Build history of the part. All positions in model axes, mm. Face numbers are marked on the shaded views. Give positions to 0.01 mm unless a question says otherwise; leave off trailing zeros. Return JSON: item names as keys, results as strings. Group by question number.
1) Drill centre lines: probe 1 along Y at (x, z) = (2.8, 3.5) (3 decimals); probe 2 along Z at (x, y) = (3.3, -1.25); probe 3 along X at (y, z) = (0, 1.5). Where is each one in solid material? Low to high. Write a range as from..to.
2) Mould opens along Y. For the marked faces 1, 2 and 3 say: released by +Y, released by -Y, zero draft, split by the parting line, or undercut.
3) Drop a flat-ended pin along its axis: pin 1 (3 mm diameter, centred on y = -2, z = 3.5, fed in from -X). Give the stop position or say it passes through.
```python
from build123d import *

# Parameters (mm, degrees)
BOSS_EXTRUDE1_DEPTH = 6.05
FILLET1_R           = 0.5
FILLET2_R           = 0.1


with BuildPart() as part:
    # Sketch1 → Boss-Extrude1 (new body)
    with BuildSketch(Plane.XY):
        with BuildLine():
            Line((2.5, -3.575), (3.203025913, -3.575))
            ThreePointArc((3.203025913, -3.575), (4.8, 0), (3.203025913, 3.575))
            Line((3.203025913, 3.575), (2.3, 3.575))
            Line((2.3, 3.575), (2.3, 2.567103802))
            ThreePointArc((2.3, 2.567103802), (3.446740769, 0), (2.3, -2.567103802))
            Line((2.3, -2.567103802), (2.5, -3.575))
        make_face()
    extrude(amount=BOSS_EXTRUDE1_DEPTH)

    # Fillet1
    fillet1_edges = [part.edges().sort_by_distance(p)[0] for p in [
        (2.751512957, 3.575, 0),
        (2.3, 2.567103802, 3.025),
        (2.3, -2.567103802, 3.025),
        (2.851512957, -3.575, 0),
        (2.851512957, -3.575, 6.05),
        (2.751512957, 3.575, 6.05),
    ]]
    fillet(fillet1_edges, radius=FILLET1_R)

    # Fillet2
    fillet2_edges = [part.edges().sort_by_distance(p)[0] for p in [
        (2.5, -3.575, 3.025),
        (3.203025913, -3.575, 3.025),
        (4.8, 0, 6.05),
        (4.8, 0, 0),
        (3.203025913, 3.575, 3.025),
        (3.383378785, 3.40481248, 5.925797449),
        (3.383378785, 3.40481248, 0.124202551),
        (3.383378797, -3.404812467, 5.92579746),
        (3.383378797, -3.404812467, 0.12420254),
        (2.376908676, -2.954683613, 0),
        (3.446633835, 0.027150287, 0),
        (2.3, 2.928251838, 0),
        (2.337743829, 2.590927621, 0),
        (2.363671694, -2.596363527, 0),
        (2.376908676, -2.954683613, 6.05),
        (2.470600688, -3.426842727, 5.905255817),
        (2.470600688, -3.426842727, 0.144744183),
        (2.3, 2.928251838, 6.05),
        (3.446633835, 0.027150287, 6.05),
        (2.337743829, 2.590927621, 6.05),
        (2.363671694, -2.596363527, 6.05),
        (2.3, 3.575, 3.025),
        (2.3, 3.428553391, 5.903553391),
        (2.3, 3.428553391, 0.146446609),
    ]]
    fillet(fillet2_edges, radius=FILLET2_R)


solid = part.part
```
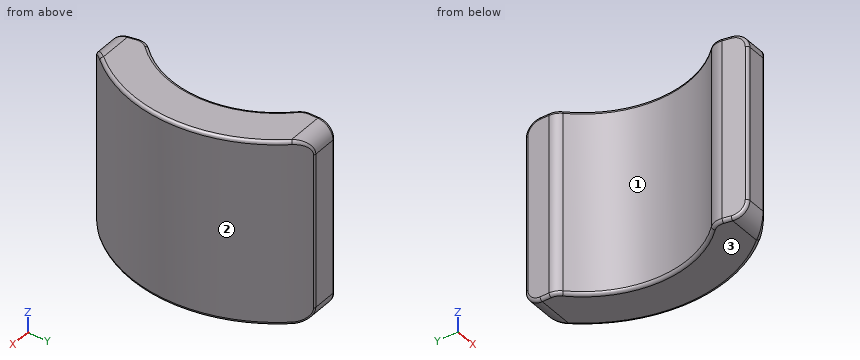
Results:
{
 "1": {"probe 1": "-3.575..-2.01, 2.01..3.575", "probe 2": "0..6.05", "probe 3": "3.45..4.8"},
 "2": {"face 1": "undercut", "face 2": "split by the parting line", "face 3": "zero draft"},
 "3": {"pin 1": "x = 2.34"}
}
